```python
from build123d import *

# Parameters (mm, degrees)
MODEL_R           = 1.4
MODEL_R_2         = 1
BRIDA_BASE1_DEPTH = 1


# Sheet-metal steps are written as plain solids
with BuildPart() as part:
    # Model → Brida base1 (new body)
    with BuildSketch(Plane.XY):
        with BuildLine():
            Line((40.2059904, -5.7615616), (42.197855138, 22.819737764))
            ThreePointArc((42.197855138, 22.819737764), (42.212695742, 22.935208537), (42.240856149, 23.048171958))
            Line((42.240856149, 23.048171958), (42.538911562, 24.003067399))
            ThreePointArc((42.538911562, 24.003067399), (42.562673339, 24.508023196), (42.336424948, 24.960081427))
            Line((42.336424948, 24.960081427), (38.453897645, 29.390683716))
            ThreePointArc((38.453897645, 29.390683716), (38.270016908, 29.697670508), (38.2059904, 30.049740987))
            Line((38.2059904, 30.049740987), (38.2059904, 46.085251303))
            ThreePointArc((38.2059904, 46.085251303), (38.498883619, 46.792358084), (39.2059904, 47.085251303))
            Line((39.2059904, 47.085251303), (41.2059904, 47.085251303))
            ThreePointArc((41.2059904, 47.085251303), (41.913097181, 46.792358084), (42.2059904, 46.085251303))
            Line((42.2059904, 46.085251303), (42.2059904, 37.778119438))
            ThreePointArc((42.2059904, 37.778119438), (42.498883619, 37.071012657), (43.2059904, 36.778119438))
            Line((43.2059904, 36.778119438), (47.2059904, 36.778119438))
            ThreePointArc((47.2059904, 36.778119438), (47.913097181, 37.071012657), (48.2059904, 37.778119438))
            Line((48.2059904, 37.778119438), (48.2059904, 46.085251303))
            ThreePointArc((48.2059904, 46.085251303), (48.498883619, 46.792358084), (49.2059904, 47.085251303))
            Line((49.2059904, 47.085251303), (51.2059904, 47.085251303))
            ThreePointArc((51.2059904, 47.085251303), (51.913097181, 46.792358084), (52.2059904, 46.085251303))
            Line((52.2059904, 46.085251303), (52.2059904, 30.049740987))
            ThreePointArc((52.2059904, 30.049740987), (52.141963892, 29.697670508), (51.958083155, 29.390683716))
            Line((51.958083155, 29.390683716), (48.075555852, 24.960081427))
            ThreePointArc((48.075555852, 24.960081427), (47.849307461, 24.508023196), (47.873069238, 24.003067399))
            Line((47.873069238, 24.003067399), (48.171124651, 23.048171958))
            ThreePointArc((48.171124651, 23.048171958), (48.199285058, 22.935208537), (48.214125662, 22.819737764))
            Line((48.214125662, 22.819737764), (50.2059904, -5.7615616))
            Line((50.2059904, -5.7615616), (50.2059904, -15.7615616))
            ThreePointArc((50.2059904, -15.7615616), (45.2059904, -20.7615616), (40.2059904, -15.7615616))
            Line((40.2059904, -15.7615616), (40.2059904, -5.7615616))
        make_face()
        with Locations((45.2059904, -15.7615616)):
            Circle(MODEL_R, mode=Mode.SUBTRACT)
        with Locations((45.2059904, -3.2615616)):
            Circle(MODEL_R_2, mode=Mode.SUBTRACT)
    extrude(amount=-BRIDA_BASE1_DEPTH)


solid = part.part
```
Here's how the part is built. I have some questions about the finished solid (model axes, mm). A direction names the side the tool comes from. Give positions to 0.01 mm unless a question says otherwise; leave off trailing zeros. Order: outer loops, then holes, each group sorted by start corner. A loop starts at its lowest first (then second) coordinate and runs counter-clockwise, first axis right, second up. Notation, with made-up numbers: M 65.25,-5 L 91.25,-5 A18 ccw 91.25,19 Z; hole C 77,75.5 d6. An arc over 180 degrees is marked long. Use a Markdown table: item, result. Add a question column.
1. Suppose I cut it at B-B (z = -0.8). Give the number of separate pieces and of enclosed holes in the cut face, and give its area (3 significant figures).
2. For pin 1 Ø6 at (x, y) = (48, 35.5) entering from +Z, with a flat end and sliding along its axis, tell me the tip position at first contact or that it passes through.
3. Suppose I cut it at C-C (y = 26). List the corners of the cut face in (x, z) for me, and give its area (3 significant figures).
4. Suppose I cut it at A-A (y = 39.5). List the corners of the cut face in (x, z) for me.
5. Suppose I cut it at D-D (y = 3.5). List the corners of the cut face in (x, z) for me, and give its area (3 significant figures).
6. If we mould it in two halves opening along X, with no side actions, what happens to faces 4 (the cylindrical face through (44.207, -3.218, -0.493)), 5 (the flat face through (40.422, 27.144, -0.493)), 6 (the flat face through (45, 14, 0))? For each: +X half, -X half, draft (parallel to the pull), parting line (faces both ways), or undercut.
7. On a 3-axis mill with a long thin cutter (end or side, diameter ignored), from which of +Z, -Z, +X, -X, +Y, -Y can I reach the whole of each face in a straight line? I mean faces 1 (the flat face through (50.044, 27.206, -0.493)), 2 (the flat face through (45, 14, -1)), 3 (the flat face through (41.19, 8.33, -0.49)). Say none if no direction works.
8. I need wall thicknesses on probe 1 along Y at (x, z) = (44.5, -0.45); probe 2 along Y at (x, z) = (46, -0.75); probe 3 along X at (y, z) = (-13, -0.05). Which ranges of each line are inside material? Lowest first, please. Write a range as from..to.
Results list:
| question | item | result |
|---|---|---|
| 1 | separate pieces | 1 |
| 1 | enclosed holes | 2 |
| 1 | area | 599 mm² |
| 2 | pin 1 | stops at z = 0 |
| 3 | outline | M 41.43,-1 L 48.99,-1 L 48.99,0 L 41.43,0 Z |
| 3 | area | 7.56 mm² |
| 4 | outline | M 38.21,-1 L 42.21,-1 L 42.21,0 L 38.21,0 Z; M 48.21,-1 L 52.21,-1 L 52.21,0 L 48.21,0 Z |
| 5 | outline | M 40.85,-1 L 49.56,-1 L 49.56,0 L 40.85,0 Z |
| 5 | area | 8.71 mm² |
| 6 | face 4 | undercut |
| 6 | face 5 | -X half |
| 6 | face 6 | draft |
| 7 | face 1 | +Z, -Z, +X |
| 7 | face 2 | -Z, +X, -X, +Y, -Y |
| 7 | face 3 | +Z, -Z, -X |
| 8 | probe 1 | y = -20.71..-16.97, -14.55..-3.97, -2.55..36.78 |
| 8 | probe 2 | y = -20.7..-16.91, -14.61..-3.87, -2.65..36.78 |
| 8 | probe 3 | x = 40.21..50.21 |
